Build history of the part. All positions in model axes, mm. Face numbers are marked on the shaded views. A direction names the side the tool comes from. Give positions to 0.01 mm unless a question says otherwise; leave off trailing zeros. Order: outer loops, then holes, each group sorted by start corner. A loop starts at its lowest first (then second) coordinate and runs counter-clockwise, first axis right, second up. Notation, with made-up numbers: (16.5, -18) - (44.5, -18) arc R11 ccw to (44.5, 1) - close; hole circle Ø9 at (75.5, 7.25). An arc over 180 degrees is marked (long way). Answer in a Markdown table with one row per item.
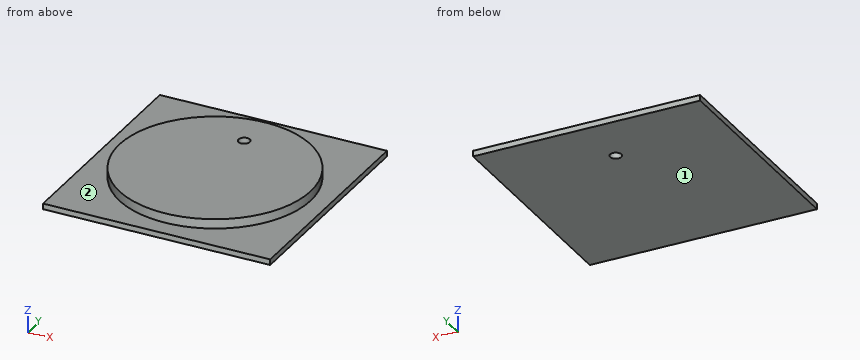
```python
from build123d import *

# Parameters (mm, degrees)
SKETCH1_R           = 25.25
BOSS_EXTRUDE1_DEPTH = 4
SKETCH1_4_W         = 60
SKETCH1_4_H         = 60
BOSS_EXTRUDE2_DEPTH = 1.5
SKETCH2_R           = 1.5
CUT_EXTRUDE1_DEPTH  = 43.614551505


with BuildPart() as part:
    # Sketch1 → Boss-Extrude1 (new body)
    with BuildSketch(Plane.XY):
        Circle(SKETCH1_R)
    extrude(amount=BOSS_EXTRUDE1_DEPTH)

    # Sketch1_4 → Boss-Extrude2 (add)
    with BuildSketch(Plane.XY):
        Rectangle(SKETCH1_4_W, SKETCH1_4_H)
    extrude(amount=BOSS_EXTRUDE2_DEPTH)

    # Sketch2 → Cut-Extrude1 (cut, through all)
    with BuildSketch(Plane.XY.offset(4)):
        with Locations((0, 15)):
            Circle(SKETCH2_R)
    extrude(amount=-CUT_EXTRUDE1_DEPTH, mode=Mode.SUBTRACT)


solid = part.part
```
1. Cut at C-C on y = 15. Write the cut outline in (x, z).
Check result:
| item | result |
|---|---|
| outline | (-30, 0) - (-1.5, 0) - (-1.5, 4) - (-20.31, 4) - (-20.31, 1.5) - (-30, 1.5) - close; (1.5, 0) - (30, 0) - (30, 1.5) - (20.31, 1.5) - (20.31, 4) - (1.5, 4) - close |
2. Probe line 1 (Y direction, x = 0, z = 1.9); line 2 (Y direction, x = 0, z = 0.95); line 3 (Z direction, x = 18.5, y = 27.5). List the from-to ranges inside material, lowest first.
Check result:
| item | result |
|---|---|
| line 1 | y = -25.25 to 13.5, 16.5 to 25.25 |
| line 2 | y = -30 to 13.5, 16.5 to 30 |
| line 3 | z = 0 to 1.5 |
3. Which spindle directions (+Z, -Z, +X, -X, +Y, -Y) get a long thin tool onto all of the face, cutting with end or side? Do the marked faces 1 and 2. Say none if no direction does.
Check result:
| item | result |
|---|---|
| face 1 | -Z, +X, -X, +Y, -Y |
| face 2 | +Z |
4. Cut at A-A on x = 0. Write the cut outline in (y, z), and give its area (3 significant figures).
Check result:
| item | result |
|---|---|
| outline | (-30, 0) - (13.5, 0) - (13.5, 4) - (-25.25, 4) - (-25.25, 1.5) - (-30, 1.5) - close; (16.5, 0) - (30, 0) - (30, 1.5) - (25.25, 1.5) - (25.25, 4) - (16.5, 4) - close |
| area | 204 mm² |
5. Cut at B-B on y = 0. Write the cut outline in (x, z), and give its area (3 significant figures).
Check result:
| item | result |
|---|---|
| outline | (-30, 0) - (30, 0) - (30, 1.5) - (25.25, 1.5) - (25.25, 4) - (-25.25, 4) - (-25.25, 1.5) - (-30, 1.5) - close |
| area | 216 mm² |
6. Cut at D-D on z = 3.4. Write the cut outline in (x, y).
Check result:
| item | result |
|---|---|
| outline | circle Ø50.5 at (0, 0); hole circle Ø3 at (0, 15) |
7. Drop flat-ended pins along their axis: P1, Ø2.5, axis at x = 0, y = 15, coming from the +Z side; P2, Ø2, axis at x = 19.5, y = -21, coming from the +Z side. Give the stop position or say it passes through.
Check result:
| item | result |
|---|---|
| P1 | passes through |
| P2 | stops at z = 1.5 |
